from build123d import *

# Parameters (mm, degrees)
ESQUISSE1_W             = 42
ESQUISSE1_H             = 62
ESQUISSE1_R             = 13.4
BOSS_EXTRU_1_DEPTH      = 8
ENL_V_MAT_EXTRU_2_REACH = 10
ESQUISSE3_W             = 42
ESQUISSE3_H             = 8
ESQUISSE2_R             = 2.2
ENL_V_MAT_EXTRU_1_DEPTH = 9


with BuildPart() as part:
    # Esquisse1 → Boss.-Extru.1 (new body)
    with BuildSketch(Plane(origin=(0, 0, 0), x_dir=(1, 0, 0), z_dir=(0, 1, 0))):
        with Locations((21, 31)):
            Rectangle(ESQUISSE1_W, ESQUISSE1_H)
        with Locations((21, 31)):
            Circle(ESQUISSE1_R, mode=Mode.SUBTRACT)
    extrude(amount=BOSS_EXTRU_1_DEPTH)

    # Esquisse3 → Enlèv. mat.-Extru.2 (cut, up to next)
    with BuildSketch(Plane(origin=(0, 8, 0), x_dir=(1, 0, 0), z_dir=(0, 1, 0)), mode=Mode.PRIVATE) as enl_v_mat_extru_2_sk1:
        with Locations((21, 58)):
            Rectangle(ESQUISSE3_W, ESQUISSE3_H)
    enl_v_mat_extru_2_tool1 = extrude(enl_v_mat_extru_2_sk1.sketch, amount=-ENL_V_MAT_EXTRU_2_REACH, mode=Mode.PRIVATE) & part.part
    add(enl_v_mat_extru_2_tool1.solids().sort_by_distance((21, 8, -58))[0], mode=Mode.SUBTRACT)

    # Esquisse2 → Enlèv. mat.-Extru.1 (cut, through all)
    with BuildSketch(Plane(origin=(0, 8, 0), x_dir=(1, 0, 0), z_dir=(0, 1, 0))):
        with Locations((9, 50)):
            Circle(ESQUISSE2_R)
        with Locations((33, 50)):
            Circle(ESQUISSE2_R)
        with Locations((33, 4)):
            Circle(ESQUISSE2_R)
        with Locations((9, 4)):
            Circle(ESQUISSE2_R)
    extrude(amount=-ENL_V_MAT_EXTRU_1_DEPTH, mode=Mode.SUBTRACT)


solid = part.part
Read the model definition and answer for the solid it produces. Units are mm, in the model's axes. Round coordinates to 2 decimals unless told otherwise and drop trailing zeros. Order: outer loops, then holes, each group sorted by start corner. A loop starts at its lowest first (then second) coordinate and runs counter-clockwise, first axis right, second up. Notation, with made-up numbers: (-3.75, 49.25) - (6.25, 49.25) arc R30 ccw to (6.25, 84.25) - close; hole circle Ø2 at (48, -25.5). An arc over 180 degrees is marked (long way). Use one line per item in the form item = value. Start each with the question number.
(1) The part is cut by section A-A (y = 5.75). Give the vertices of the cut face in (x, z).
(2) A flat-ended cylindrical pin translates along its axis: pin 1 Ø3.5 at (x, z) = (33, -50) entering from -Y. Find the tip coordinate at first contact, or state that the pin passes through.
(3) The part is cut by section D-D (z = -29). Give the vertices of the cut face in (x, y), then the cut area to 3 significant figures.
(4) Determine the mould class of faces 1 (the face through (21, 4, 0)), 2 (the face through (8.523, 4.056, -47.852)), 3 (the face through (11, 0, -21)) for opening direction Z: +Z half, -Z half, draft (parallel to the pull), parting line (faces both ways), or undercut.
(5) Find the intervals of material crossed by line 1 along X through (y, z) = (4.75, -50); line 2 along X through (y, z) = (4, -31); line 3 along Z through (x, y) = (33, 6), in increasing order. Write a range as from..to.
(6) The part is cut by section C-C (z = -50). Give the vertices of the cut face in (x, y).
(7) The part is cut by section B-B (x = 21). Give the vertices of the cut face in (y, z).
Checked values:
q1.outline = (0, -54) - (42, -54) - (42, 0) - (0, 0) - close; hole circle Ø4.4 at (9, -50); hole circle Ø4.4 at (9, -4); hole circle Ø26.8 at (21, -31); hole circle Ø4.4 at (33, -50); hole circle Ø4.4 at (33, -4)
q2.pin_1 = through
q3.outline = (0, 0) - (7.75, 0) - (7.75, 8) - (0, 8) - close; (34.25, 0) - (42, 0) - (42, 8) - (34.25, 8) - close
q3.area = 124 mm^2
q4.face_1 = +Z half
q4.face_2 = undercut
q4.face_3 = draft
q5.line_1 = 0..6.8, 11.2..30.8, 35.2..42
q5.line_2 = 0..7.6, 34.4..42
q5.line_3 = -54..-52.2, -47.8..-36.96, -25.04..-6.2, -1.8..0
q6.outline = (0, 0) - (6.8, 0) - (6.8, 8) - (0, 8) - close; (11.2, 0) - (30.8, 0) - (30.8, 8) - (11.2, 8) - close; (35.2, 0) - (42, 0) - (42, 8) - (35.2, 8) - close
q7.outline = (0, -54) - (8, -54) - (8, -44.4) - (0, -44.4) - close; (0, -17.6) - (8, -17.6) - (8, 0) - (0, 0) - close
